Geometry check sheet. Reference: the model listing, model coordinates, mm. A direction names the side the tool comes from. Coordinates: 2 decimals unless noted, no trailing zeros. Write each loop counter-clockwise with the first axis right and the second up, starting at its lowest first coordinate (ties: lowest second). Pieces come first, ordered by that corner, then holes. Notation, with made-up numbers: (44.5, 14) -> (103.5, 14) arc R20 ccw to (103.5, 40) -> close; hole circle Ø7 at (9, 83.25). An arc over 180 degrees is marked (long way). One line per question, with ' | ' between items.
from build123d import *

# Parameters (mm, degrees)
F1_DEPTH  = 57.15
F3_DEPTH  = 25.4
F5_DEPTH  = 3.81
F7_DEPTH  = 3.81
F8_R      = 2.0828
F9_DEPTH  = 12.7
F8_R_2    = 2.1082
F10_DEPTH = 43.816
F8_R_3    = 3.556
F11_DEPTH = 9.652


with BuildPart() as f1:
    # F0 (on Right) → F1 (new body)
    with BuildSketch(Plane.YZ):
        Polygon((0, 11.176), (0, 0), (25.4, 0), (25.4, 11.176), (20.6375, 11.176), (20.6375, 43.815), (4.7625, 43.815), (4.7625, 11.176), align=None)
    extrude(amount=-F1_DEPTH)

    # F2 (on face) → F3 (cut)
    with BuildSketch(Plane.XZ.offset(-4.7625)):
        with BuildLine():
            Line((-12.7, 43.815), (-44.45, 43.815))
            Line((-44.45, 43.815), (-44.45, 38.989))
            ThreePointArc((-44.45, 38.989), (-43.036497, 35.576503), (-39.624, 34.163))
            Line((-39.624, 34.163), (-17.526, 34.163))
            ThreePointArc((-17.526, 34.163), (-14.113503, 35.576503), (-12.7, 38.989))
            Line((-12.7, 38.989), (-12.7, 43.815))
        make_face()
    extrude(amount=-F3_DEPTH, mode=Mode.SUBTRACT)

    # F4 (on face) → F5 (cut)
    with BuildSketch(Plane.XZ.offset(-4.7625)):
        with BuildLine():
            Line((-15.875, 29.0322), (-41.275, 29.0322))
            ThreePointArc((-41.275, 29.0322), (-44.687497, 27.618697), (-46.101, 24.2062))
            Line((-46.101, 24.2062), (-46.101, 21.1582))
            ThreePointArc((-46.101, 21.1582), (-44.687497, 17.745703), (-41.275, 16.3322))
            Line((-41.275, 16.3322), (-15.875, 16.3322))
            ThreePointArc((-15.875, 16.3322), (-12.462503, 17.745703), (-11.049, 21.1582))
            Line((-11.049, 21.1582), (-11.049, 24.2062))
            ThreePointArc((-11.049, 24.2062), (-12.462503, 27.618697), (-15.875, 29.0322))
        make_face()
    extrude(amount=-F5_DEPTH, mode=Mode.SUBTRACT)

    # F6 (on face) → F7 (cut)
    with BuildSketch(Plane(origin=(0, 20.6375, 0), x_dir=(-1, 0, 0), z_dir=(0, 1, 0))):
        with BuildLine():
            Line((41.275, 29.0322), (15.875, 29.0322))
            ThreePointArc((15.875, 29.0322), (12.462503, 27.618697), (11.049, 24.2062))
            Line((11.049, 24.2062), (11.049, 21.1582))
            ThreePointArc((11.049, 21.1582), (12.462503, 17.745703), (15.875, 16.3322))
            Line((15.875, 16.3322), (41.275, 16.3322))
            ThreePointArc((41.275, 16.3322), (44.687497, 17.745703), (46.101, 21.1582))
            Line((46.101, 21.1582), (46.101, 24.2062))
            ThreePointArc((46.101, 24.2062), (44.687497, 27.618697), (41.275, 29.0322))
        make_face()
    extrude(amount=-F7_DEPTH, mode=Mode.SUBTRACT)

    # F8 (on face) → F9 (cut)
    with BuildSketch(Plane(origin=(0, 0, 0), x_dir=(1, 0, 0), z_dir=(0, 0, -1))):
        with Locations((-44.45, -12.7)):
            Circle(F8_R)
        with Locations((-12.7, -12.7)):
            Circle(F8_R)
    extrude(amount=-F9_DEPTH, mode=Mode.SUBTRACT)

    # F8 (on face) → F10 (cut, through all)
    with BuildSketch(Plane(origin=(0, 0, 0), x_dir=(1, 0, 0), z_dir=(0, 0, -1))):
        with Locations((-51.562, -12.7)):
            Circle(F8_R_2)
        with Locations((-5.588, -12.7)):
            Circle(F8_R_2)
    extrude(amount=-F10_DEPTH, mode=Mode.SUBTRACT)

    # F8 (on face) → F11 (cut)
    with BuildSketch(Plane(origin=(0, 0, 0), x_dir=(1, 0, 0), z_dir=(0, 0, -1))):
        with Locations((-51.562, -12.7)):
            Circle(F8_R_3)
        with Locations((-51.562, -12.7)):
            Circle(F8_R_2, mode=Mode.SUBTRACT)
        with Locations((-5.588, -12.7)):
            Circle(F8_R_3)
        with Locations((-5.588, -12.7)):
            Circle(F8_R_2, mode=Mode.SUBTRACT)
    extrude(amount=-F11_DEPTH, mode=Mode.SUBTRACT)


solid = f1.part
1. Mould release check, pull along X, two halves, no side actions. Record for faces 1 (the face through (-28, 2, 11.176)), 2 (the face through (0, 13, 17)), 3 (the face through (-28, 16.828, 23)): released by +X, released by -X, zero draft, split by the parting line, or undercut.
Worked answers:
face 1: zero draft | face 2: released by +X | face 3: undercut
2. Cross-section at D-D on z = 33.5. Record the boundary of the cut face in (x, y), and give its area (3 significant figures).
Worked answers:
outline: (-57.15, 4.76) -> (0, 4.76) -> (0, 20.64) -> (-57.15, 20.64) -> close; hole circle Ø4.22 at (-51.56, 12.7); hole circle Ø4.22 at (-5.59, 12.7) | area: 879 mm²
3. Cross-section at A-A on y = 12.7. Give the number of separate pieces and of enclosed holes in the cut face, and give its area (3 significant figures).
Worked answers:
separate pieces: 3 | enclosed holes: 0 | area: 1,680 mm²
4. Cross-section at B-B on z = 7.5. Record the boundary of the cut face in (x, y), and give its area (3 significant figures).
Worked answers:
outline: (-57.15, 0) -> (0, 0) -> (0, 25.4) -> (-57.15, 25.4) -> close; hole circle Ø7.11 at (-51.56, 12.7); hole circle Ø4.17 at (-44.45, 12.7); hole circle Ø4.17 at (-12.7, 12.7); hole circle Ø7.11 at (-5.59, 12.7) | area: 1,340 mm²
5. Cross-section at C-C on x = -35. Record the boundary of the cut face in (y, z), and give its area (3 significant figures).
Worked answers:
outline: (0, 0) -> (25.4, 0) -> (25.4, 11.18) -> (20.64, 11.18) -> (20.64, 16.33) -> (16.83, 16.33) -> (16.83, 29.03) -> (20.64, 29.03) -> (20.64, 34.16) -> (4.76, 34.16) -> (4.76, 29.03) -> (8.57, 29.03) -> (8.57, 16.33) -> (4.76, 16.33) -> (4.76, 11.18) -> (0, 11.18) -> close | area: 552 mm²
6. Go/stop test with flat-tipped pins: P1, Ø4, axis at x = -23, y = 19, coming from the +Z side; P2, Ø4, axis at x = -16, y = 23.5, coming from the +Z side; P3, Ø2, axis at x = -13.5, z = 12.5, coming from the +Y side. Record where each tip stops, or that it passes through.
Worked answers:
P1: z = 34.16 | P2: z = 11.18 | P3: y = 20.64
7. Material ranges on line 1 (X direction, y = 12.7, z = 3.5); line 2 (X direction, y = 12.7, z = 28.5); line 3 (Z direction, x = -24.5, y = 8.25), recorded low to high. Write a range as from..to.
Worked answers:
line 1: -57.15..-55.12, -48.01..-46.53, -42.37..-14.78, -10.62..-9.14, -2.03..0 | line 2: -57.15..-53.67, -49.45..-7.7, -3.48..0 | line 3: 0..16.33, 29.03..34.16
8. Tool access check on faces 4 (the face through (-44.725, 18.759, 27.581)), 5 (the face through (-14.15, 12.59, 35.54)), 6 (the face through (-46.101, 7, 23)), 7 (the face through (-49, 13, 9.652)). Record the directions out of +Z, -Z, +X, -X, +Y, -Y that give a thin tool (end or side, any length) a straight path to the whole face; none if there is none.
Worked answers:
face 4: +Y | face 5: +Z, +Y, -Y | face 6: -Y | face 7: -Z
